Autodesk Inventor part; units mm, degrees
ref_plane "YZ Plane" through (0, 0, 0) normal (1, 0, 0) x (0, 1, 0)
ref_plane "XZ Plane" through (0, 0, 0) normal (0, 1, 0) x (-1, 0, 0)
ref_plane "XY Plane" through (0, 0, 0) normal (0, 0, 1) x (1, 0, 0)
sketch "Sketch1" plane through (0, 0, 0) normal (0, 0, 1) x (1, 0, 0)
  circle A0 centre (0, 0) radius 40
  dimension "d0" = 80
extrude "Extrusion1" add sketch "Sketch1" along normal blind 6
sketch "Sketch2" plane through (0, 0, 6) normal (0, 0, 1) x (1, 0, 0)
  circle A0 centre (0, 24) radius 4
  point P0 (0, 0)
  dimension "d3" = 8
  dimension "d4" = 24
extrude "Extrusion2" add sketch "Sketch2" along normal blind 7.5
sketch "Sketch3" plane through (0, 0, 6) normal (0, 0, 1) x (1, 0, 0)
  line L0 (0, 0) -> (0, 40) construction
  circle A0 centre (0, 0) radius 40 construction
ref_plane "Work Plane1" through (0, 40, 6) normal (0, 1, 0) x (-1, 0, 0)
sketch "Sketch4" plane through (0, 40, 6) normal (0, 1, 0) x (-1, 0, 0)
  line L0 (-4.5029, 7.5) -> (4.4959, 7.5)
  line L1 (4, 7.5) -> (-4, 7.5)
  line L2 (-4, 0) -> (-4, 7.5)
  line L3 (4, 7.5) -> (4, 4.5)
  line L4 (4, 4.5) -> (-4, 7.5)
  point P0 (0, -6)
  dimension "d12" = 3
extrude "Extrusion3" cut sketch "Sketch4" against normal blind 25
pattern_circular "Circular Pattern1" count 4 over 360 about axis through (0, 0, 0) along (0, 0, 1) of "Extrusion2", "Extrusion3"
sketch "Sketch5" plane through (0, 0, 0) normal (0, 0, -1) x (-1, 0, 0)
  circle A0 centre (0, 0) radius 6
  dimension "d13" = 12
extrude "Extrusion4" add sketch "Sketch5" along normal blind 2
properties part number "innerbaycon4"
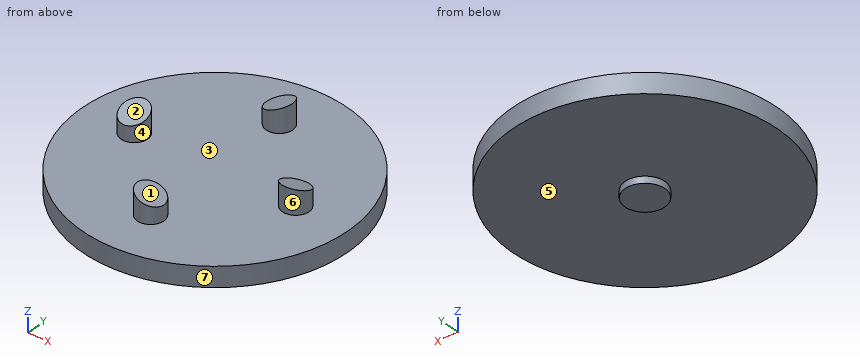
Geometry check sheet. Reference: the model listing, model coordinates, mm. Face numbers are marked on the shaded views. A direction names the side the tool comes from. Round coordinates to 2 decimals unless told otherwise and drop trailing zeros. Order: outer loops, then holes, each group sorted by start corner. A loop starts at its lowest first (then second) coordinate and runs counter-clockwise, first axis right, second up. Notation, with made-up numbers: (13, 51) - (42, 51) arc R27 ccw to (42, 70) - close; hole circle Ø9 at (-0.75, 10.25). An arc over 180 degrees is marked (long way). Use a Markdown table: item, result. Add a question column.
(1) Sectioned sample at D-D, the plane x = 24. Enter the section's corners in (y, z).
(2) Material ranges on line 1 along Z through (x, y) = (7.5, 28.5); line 2 along X through (y, z) = (27.5, 1.75); line 3 along Y through (x, z) = (24, 6.5), recorded low to high. Write a range as [from, to].
(3) Sectioned sample at B-B, the plane z = 11.5. Enter the section's corners in (x, y).
(4) Depth check by flat-ended pin: pin 1 (2 mm diameter, centred on x = -20, y = 22.5, fed in from -Z); pin 2 (1.5 mm diameter, centred on x = -8, z = 4.5, fed in from +Y); pin 3 (5 mm diameter, centred on y = 10, z = 5.5, fed in from +X). Enter the tip coordinate at first touch or a pass-through.
(5) Sectioned sample at A-A, the plane x = 0. Enter the section's corners in (y, z).
(6) Release check for a two-part mould opening along X. For the marked faces 4, 5, 6 and 7 record: pulls with the +X half, pulls with the -X half, needs draft (parallel to the pull), parting line crosses it, or undercut.
(7) Tool access check on the marked faces 1, 2 and 3. Record the directions out of +Z, -Z, +X, -X, +Y, -Y that give a thin tool (end or side, any length) a straight path to the whole face; none if there is none.
Answers below:
| question | item | result |
|---|---|---|
| 1 | outline | (-32, 0) - (32, 0) - (32, 6) - (4, 6) - (4, 10.5) - (-4, 13.5) - (-4, 6) - (-32, 6) - close |
| 2 | line 1 | [0, 6] |
| 2 | line 2 | [-29.05, 29.05] |
| 2 | line 3 | [-4, 4] |
| 3 | outline | (-27.77, -1.33) - (-20.23, -1.33) arc R4 ccw (long way) to start; (-1.33, 20.23) arc R4 ccw (long way) to (-1.33, 27.77) - close; (1.33, -27.77) - (1.33, -20.23) arc R4 ccw (long way) to start; (20.23, 1.33) arc R4 ccw (long way) to (27.77, 1.33) - close |
| 4 | pin 1 | z = 0 |
| 4 | pin 2 | y = 39.34 |
| 4 | pin 3 | x = 39.29 |
| 5 | outline | (-40, 0) - (-6, 0) - (-6, -2) - (6, -2) - (6, 0) - (40, 0) - (40, 6) - (28, 6) - (28, 12) - (20, 12) - (20, 6) - (-20, 6) - (-20, 12) - (-28, 12) - (-28, 6) - (-40, 6) - close |
| 6 | face 4 | undercut |
| 6 | face 5 | needs draft |
| 6 | face 6 | undercut |
| 6 | face 7 | parting line crosses it |
| 7 | face 1 | +Z, +X, -Y |
| 7 | face 2 | +Z, -X, -Y |
| 7 | face 3 | +Z |
